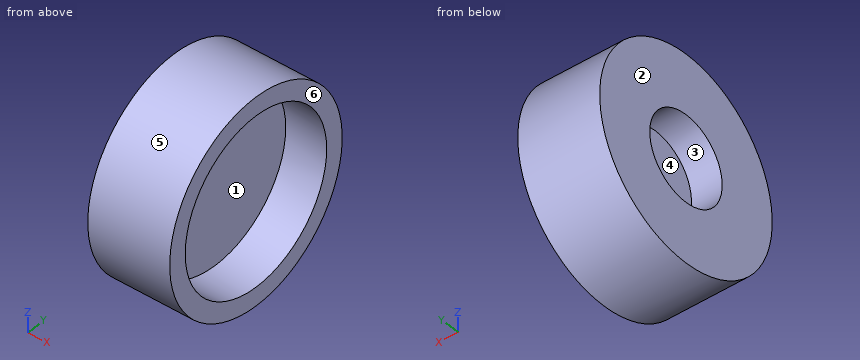
```python
from build123d import *

# Parameters (mm, degrees)
SKETCH1_R           = 5
SKETCH1_R_2         = 4.1
BOSS_EXTRUDE1_DEPTH = 4
SKETCH2_R           = 4.1
SKETCH2_R_2         = 2.1
BOSS_EXTRUDE2_DEPTH = 2
BOSS_EXTRUDE3_START = -0.5
SKETCH3_R           = 2.1
BOSS_EXTRUDE3_DEPTH = 0.5


with BuildPart() as part:
    # Sketch1 → Boss-Extrude1 (new body)
    with BuildSketch(Plane(origin=(0, 0, 0), x_dir=(0, 0, -1), z_dir=(1, 0, 0))):
        Circle(SKETCH1_R)
        Circle(SKETCH1_R_2, mode=Mode.SUBTRACT)
    extrude(amount=BOSS_EXTRUDE1_DEPTH)

    # Sketch2 → Boss-Extrude2 (add)
    with BuildSketch(Plane.ZY):
        Circle(SKETCH2_R)
        Circle(SKETCH2_R_2, mode=Mode.SUBTRACT)
    extrude(amount=-BOSS_EXTRUDE2_DEPTH)

    # Sketch3 → Boss-Extrude3 (add)
    with BuildSketch(Plane(origin=(2, 0, 0), x_dir=(0, 0, -1), z_dir=(1, 0, 0)).offset(BOSS_EXTRUDE3_START)):
        with Locations(Location((0, 0, 0), (0, 0, 180))):
            Circle(SKETCH3_R)
    extrude(amount=BOSS_EXTRUDE3_DEPTH)


solid = part.part
```
Can you work these out from the model? Positions are in its coordinate system, mm. Face numbers are marked on the shaded views. A direction names the side the tool comes from. Coordinates: 2 decimals unless noted, no trailing zeros. Order: outer loops, then holes, each group sorted by start corner. A loop starts at its lowest first (then second) coordinate and runs counter-clockwise, first axis right, second up. Notation, with made-up numbers: (-28.75, 12) - (-0.75, 12) arc R17 ccw to (-0.75, 35) - close; hole circle Ø1 at (76.25, 54.25). An arc over 180 degrees is marked (long way). Answer in a Markdown table with one row per item.
1. Suppose I cut it at A-A (y = 0). Please give me the cut outline in (x, z).
Reply:
| item | result |
|---|---|
| outline | (0, -5) - (4, -5) - (4, -4.1) - (2, -4.1) - (2, 4.1) - (4, 4.1) - (4, 5) - (0, 5) - (0, 2.1) - (1.5, 2.1) - (1.5, -2.1) - (0, -2.1) - close |
2. For pin 1 (1 mm diameter, centred on x = 3.5, y = -3.5, fed in from +Z); pin 2 (4 mm diameter, centred on y = -0.5, z = 2, fed in from +X), each with a flat end and sliding along its axis, tell me the tip position at first contact or that it passes through.
Reply:
| item | result |
|---|---|
| pin 1 | stops at z = 4 |
| pin 2 | stops at x = 2 |
3. If we mould it in two halves opening along Z, with no side actions, what happens to the marked faces 4, 5 and 6? For each: pulls with the +Z half, pulls with the -Z half, needs draft (parallel to the pull), parting line crosses it, or undercut.
Reply:
| item | result |
|---|---|
| face 4 | undercut |
| face 5 | parting line crosses it |
| face 6 | needs draft |
4. For the marked faces 1, 2 and 3, which set-ups out of +Z, -Z, +X, -X, +Y, -Y let a thin tool reach every point of the face, with its end or its side?
Reply:
| item | result |
|---|---|
| face 1 | +X |
| face 2 | +Z, -Z, -X, +Y, -Y |
| face 3 | -X |
5. Suppose I cut it at C-C (x = 3.4). Please give me the cut outline in (y, z), and give its area (3 significant figures).
Reply:
| item | result |
|---|---|
| outline | circle Ø10 at (0, 0); hole circle Ø8.2 at (0, 0) |
| area | 25.7 mm^2 |
6. If I drill on line 1 along Y through (x, z) = (1.05, 0); line 2 along X through (y, z) = (0.5, 1); line 3 along X through (y, z) = (-0.25, -4), over which ranges is the centre line in solid material (lowest first)?
Reply:
| item | result |
|---|---|
| line 1 | y = -5 to -2.1, 2.1 to 5 |
| line 2 | x = 1.5 to 2 |
| line 3 | x = 0 to 2 |
7. Suppose I cut it at D-D (z = -3). Please give me the cut outline in (x, y).
Reply:
| item | result |
|---|---|
| outline | (0, -4) - (4, -4) - (4, -2.79) - (2, -2.79) - (2, 2.79) - (4, 2.79) - (4, 4) - (0, 4) - close |
